Autodesk Inventor part; units mm, degrees
ref_plane "Pracovní rovina1" through (0, 0, 0) normal (0.2588, 0, 0.9659) x (0, 1, 0)
ref_plane "YZ Plane" through (0, 0, 0) normal (1, 0, 0) x (0, 1, 0)
ref_plane "XZ Plane" through (0, 0, 0) normal (0, 1, 0) x (-1, 0, 0)
sketch "Náčrt1" plane through (0, 0, 0) normal (0, 1, 0) x (-1, 0, 0)
  circle A0 centre (0, 0) radius 2
  circle A1 centre (0, 0) radius 12.5
  line L0 (6.7396, 10.5275) -> (-16.566, 25.4475)
  line L1 (-16.566, 25.4475) -> (-16.566, -24.5525)
  line L2 (-16.566, -24.5525) -> (6.4433, -10.7114)
  line L3 (-16.566, 25.4475) -> (-20.566, 25.4475)
  line L4 (-20.566, 25.4475) -> (-20.566, -24.5525)
  line L5 (-20.566, -24.5525) -> (-16.566, -24.5525)
  line L6 (-16.566, -24.5525) -> (-16.566, 25.4475)
  dimension "d0" = 4
  dimension "d1" = 25
  dimension "d2" = 50
  dimension "d3" = 4
extrude "Vysunutí1" add sketch "Náčrt1" along normal blind 4
sketch "Náčrt2" plane through (0, 4, 0) normal (0, 1, 0) x (1, 0, 0)
  line L0 (20.566, 24.5525) -> (16.566, 24.5525)
  line L1 (20.566, -25.4475) -> (20.566, 24.5525)
  line L2 (16.566, 24.5525) -> (20.566, 24.5525)
  line L3 (20.566, 24.5525) -> (20.566, -25.4475)
  line L4 (20.566, -25.4475) -> (16.566, -25.4475)
  line L5 (16.566, -25.4475) -> (16.566, 24.5525)
  point P0 (0, 0)
extrude "Vysunutí2" add sketch "Náčrt2" along normal blind 35
sketch "Náčrt3" plane through (20.566, 0, 25.4475) normal (1, 0, 0) x (0, 0, -1)
  circle A0 centre (13.6975, 26) radius 9.25
  circle A1 centre (37.1975, 26) radius 9.25
  line L0 (0, 39) -> (50, 39)
  line L1 (25.4475, 0) -> (25.4475, 39)
  line L2 (50, 39) -> (0, 39)
  line L3 (20.4475, 15.5) -> (30.4475, 15.5)
  line L4 (20.4475, 15.5) -> (12.1796, 16.8754)
  line L5 (30.4475, 15.5) -> (38.7155, 16.8754)
  line L6 (20.4475, 36.5) -> (30.4475, 36.5)
  line L7 (20.4475, 36.5) -> (12.1796, 35.1246)
  line L8 (30.4475, 36.5) -> (38.7155, 35.1246)
  dimension "d8" = 18.5
  dimension "d9" = 23.5
  dimension "d10" = 13
  dimension "d11" = 13
  dimension "d12" = 11.75
  dimension "d13" = 10
  dimension "d14" = 5
  dimension "d15" = 10.5
  dimension "d16" = 18.5
  dimension "d17" = 10
  dimension "d18" = 5
  dimension "d19" = 10.5
extrude "Vysunutí3" cut sketch "Náčrt3" against normal blind 35
sketch "Náčrt4" plane through (0, 0, 0) normal (0, -1, 0) x (1, 0, 0)
  circle A0 centre (0, 0) radius 2
  circle A1 centre (0, 0) radius 12.5
extrude "Vysunutí4" add sketch "Náčrt4" along normal blind 7
sketch "Náčrt5" plane through (0, 4, 0) normal (0, 1, 0) x (1, 0, 0)
  line L0 (16.566, 24.5525) -> (-6.4433, 10.7114)
  line L1 (9.566, 20.3417) -> (9.566, 15.3417)
  line L2 (-6.7396, -10.5275) -> (16.566, -25.4475)
  line L3 (9.566, -20.9662) -> (9.566, -15.9662)
  line L4 (9.566, -15.9662) -> (16.566, -20.4475)
  line L5 (16.566, -25.4475) -> (16.566, 24.5525)
  line L6 (9.566, 15.3417) -> (16.566, 19.5525)
  line L7 (16.566, 24.5525) -> (16.566, -25.4475)
  point P0 (0, 0)
  dimension "d24" = 5
  dimension "d25" = 5
  dimension "d30" = 7
  dimension "d31" = 7
extrude "Vysunutí5" add sketch "Náčrt5" along normal blind 10
chamfer "Zkosení1" distance 6.75 distance2 10 1 edges at (9.566, 14, 18.4662) measured on face at (11.8993, 14, 19.1266)
chamfer "Zkosení2" distance 6.75 distance2 10 1 edges at (9.566, 14, -17.8417) measured on face at (11.8993, 14, -18.4119)
ref_plane "Pracovní rovina1" through (0, 0, 0) normal (0.2588, 0, 0.9659) x (0, 1, 0)
sketch "Náčrt6" plane through (0, -7, 0) normal (0, -1, 0) x (1, 0, 0)
  point P0 (0, 0)
sketch "Náčrt7" plane through (0, 0, 0) normal (0.2588, 0, 0.9659) x (0, 1, 0)
  line L0 (-0.9378, 0) -> (-7, -3.5)
  line L1 (-7, -3.5) -> (-7, 3.5)
  line L2 (-7, 3.5) -> (-0.9378, 0)
  line L3 (-7, 12.5) -> (-7, -12.5)
  line L4 (0, 3.4515) -> (4, 3.4515)
  line L5 (0, 9.2347) -> (0, 3.4515)
  line L6 (0, 9.2347) -> (4, 9.2347)
  line L7 (4, 3.4515) -> (4, 9.2347)
  point P0 (0, 0)
  point P1 (-4.9793, 0)
  point P2 (-7, 0)
  point P3 (-7, 0)
  dimension "d39" = 7
extrude "Vysunutí6" cut sketch "Náčrt7" against normal blind 18.5 contours L0 L1 L2
pattern_circular "Kruhové pole1" count 12 over 360 about axis through (0, -10, 0) along (0, 1, 0) of "Vysunutí6"
properties part number "drzak"
Geometry check sheet. Reference: the model listing, model coordinates, mm. A direction names the side the tool comes from. Coordinates: 2 decimals unless noted, no trailing zeros. Order: outer loops, then holes, each group sorted by start corner. A loop starts at its lowest first (then second) coordinate and runs counter-clockwise, first axis right, second up. Notation, with made-up numbers: M 50.5,-21.75 L 76.5,-21.75 A15 cw 76.5,-8.75 Z; hole C 17,22 d11. An arc over 180 degrees is marked long. Use CSV: the item, a comma, the result in double quotes.
Item 1: Cross-section at B-B on y = 30.5. Record the cut outline in (x, z).
Returned:
outline,"M 16.57,-24.55 L 20.57,-24.55 L 20.57,-19.83 L 16.57,-19.83 Z; M 16.57,19.83 L 20.57,19.83 L 20.57,25.45 L 16.57,25.45 Z"
Item 2: Cross-section at C-C on z = 7. Record the cut outline in (x, y), then the cut area to 3 significant figures.
Returned:
outline,"M -10.36,-5.05 L -7,-0.94 L -4.04,-4.56 L -1.88,-0.94 L 0,-4.08 L 1.88,-0.94 L 4.04,-4.56 L 7,-0.94 L 10.36,-5.05 L 10.36,0 L 20.57,0 L 20.57,15.83 L 16.57,15.83 L 16.57,4 L -10.36,4 Z; M 16.57,36.17 L 20.57,36.17 L 20.57,39 L 16.57,39 Z"
area,"240 mm2"
Item 3: Thickness scan on line 1 along X through (y, z) = (2.3, 0); line 2 along X through (y, z) = (-1.25, 0); line 3 along Y through (x, z) = (18, 4). Record the ranges inside material, lowest first.
Returned:
line 1,"x = -12.5 to -2, 2 to 20.57"
line 2,"x = -12.5 to -2, 2 to 12.5"
line 3,"y = 0 to 15.5, 36.5 to 39"
Item 4: Gauge pin test, flat ends, axial feed: pin 1 Ø12 at (x, y) = (7.5, 6) entering from -Z; pin 2 Ø6 at (x, z) = (5, 9) entering from +Y; pin 3 Ø3 at (x, y) = (9, 2) entering from -Z; pin 4 Ø6 at (x, z) = (16.5, -11) entering from +Y. Record the tip position at first contact, or that the pin passes through.
Returned:
pin 1,"stops at z = -22.71"
pin 2,"stops at y = 4"
pin 3,"stops at z = -20.9"
pin 4,"stops at y = 39"
Item 5: Cross-section at D-D on y = 7.5. Record the cut outline in (x, z).
Returned:
outline,"M 11.93,-21.76 L 16.57,-24.55 L 20.57,-24.55 L 20.57,25.45 L 16.57,25.45 L 11.93,22.48 L 11.93,17.48 L 16.57,20.45 L 16.57,-19.55 L 11.93,-16.76 Z"
Item 6: Mould release check, pull along Z, two halves, no side actions. Record for faces 1 (the flat face through (8.353, -3.078, -0.959)), 2 (the cylindrical face through (-12.488, -1.197, -0.55)), 3 (the flat face through (20.566, 15, 1)): pulls with the +Z half, pulls with the -Z half, needs draft (parallel to the pull), parting line crosses it, or undercut.
Returned:
face 1,"undercut"
face 2,"parting line crosses it"
face 3,"needs draft"
Item 7: Tool access check on faces 4 (the flat face through (12.894, 8.93, -19.935)), 5 (the flat face through (19, 36.5, 0)). Record the directions out of +Z, -Z, +X, -X, +Y, -Y that give a thin tool (end or side, any length) a straight path to the whole face; none if there is none.
Returned:
face 4,"+Z, -Z, -X, +Y"
face 5,"+X, -X"
Item 8: Cross-section at A-A on x = 18.5. Record the cut outline in (y, z), then the cut area to 3 significant figures.
Returned:
outline,"M 0,-24.55 L 39,-24.55 L 39,25.45 L 0,25.45 Z; hole M 15.5,-5 L 16.88,-13.27 A9.25 ccw 35.12,-13.27 L 36.5,-5 L 36.5,5 L 35.12,13.27 A9.25 ccw 16.88,13.27 L 15.5,5 Z"
area,"1,200 mm2"
